Autodesk Inventor part; units mm, degrees
ref_plane "YZ Plane" through (0, 0, 0) normal (1, 0, 0) x (0, 1, 0)
ref_plane "XZ Plane" through (0, 0, 0) normal (0, 1, 0) x (-1, 0, 0)
ref_plane "XY Plane" through (0, 0, 0) normal (0, 0, 1) x (1, 0, 0)
sketch "Sketch1" plane through (0, 0, 0) normal (0, 1, 0) x (-1, 0, 0)
  line L0 (0, 0) -> (-76.2, 0)
  line L1 (-76.2, 0) -> (-76.2, -38.1)
  line L2 (-76.2, -38.1) -> (0, -38.1)
  line L3 (0, -38.1) -> (0, 0)
  dimension "d0" = 76.2
  dimension "d1" = 38.1
extrude "Extrusion1" add sketch "Sketch1" along normal blind 2.54
sketch "Sketch2" plane through (0, 2.54, 0) normal (0, 1, 0) x (1, 0, 0)
  line L0 (0, 0) -> (6.35, 0)
  line L1 (0, 0) -> (76.2, 0)
  line L2 (6.35, 0) -> (6.35, 38.1)
  line L3 (76.2, 38.1) -> (0, 38.1)
  line L4 (6.35, 0) -> (6.35, 9.525)
  line L5 (6.35, 38.1) -> (6.35, 28.575)
  dimension "d4" = 6.35
  dimension "d5" = 9.525
  dimension "d6" = 9.525
hole "Hole1" at (6.35, 2.54, -9.525) at (6.35, 2.54, -28.575) direction (0, -1, 0) diameter 5.08 end through all
fillet "Fillet1" radius 1.27 2 edges at (76.2, 2.54, -19.05) (76.2, 0, -19.05)
fillet "Fillet2" radius 1.27 1 edges at (0, 2.54, -19.05)
properties part number "Cover"
Verification items for the finished model (mm, model axes). Coordinates: 2 decimals unless noted, no trailing zeros. Order: outer loops, then holes, each group sorted by start corner. A loop starts at its lowest first (then second) coordinate and runs counter-clockwise, first axis right, second up. Notation, with made-up numbers: (31.5, 23.5) -> (72.5, 23.5) arc R16 ccw to (72.5, 35.5) -> close; hole circle Ø2 at (-11, -25.75). An arc over 180 degrees is marked (long way). Put each result on its own line as item: value. Start each with the question number.
1) Cross-section at A-A (x = 6.35). Enter the section's corners in (y, z) (3 decimals), plus the area to 3 significant figures.
2) Cross-section at C-C (y = 0.8). Enter the section's corners in (x, z) (3 decimals).
3) Material ranges on L1, parallel to Z at x = 6.35, y = 1.15 (3 decimals); L2, parallel to X at y = 1.35, z = -28.5; L3, parallel to X at y = 1.4, z = -17, recorded low to high.
4) Release check for a two-part mould opening along Z. For faces 1 (the cylindrical face through (7.323, 1.252, -26.229)), 2 (the flat face through (38, 0, -19)), 3 (the flat face through (39, 1, -38.1)), 4 (the flat face through (38, 1, 0)) record: pulls with the +Z half, pulls with the -Z half, needs draft (parallel to the pull), parting line crosses it, or undercut.
Geometry check:
1. outline: (0, -38.1) -> (2.54, -38.1) -> (2.54, -31.115) -> (0, -31.115) -> close; (0, -26.035) -> (2.54, -26.035) -> (2.54, -12.065) -> (0, -12.065) -> close; (0, -6.985) -> (2.54, -6.985) -> (2.54, 0) -> (0, 0) -> close
1. area: 71.0 mm^2
2. outline: (0, -38.1) -> (76.11, -38.1) -> (76.11, 0) -> (0, 0) -> close; hole circle Ø5.08 at (6.35, -28.575); hole circle Ø5.08 at (6.35, -9.525)
3. L1: z = -38.1 to -31.115, -26.035 to -12.065, -6.985 to 0
3. L2: x = 0 to 3.81, 8.89 to 76.2
3. L3: x = 0.01 to 76.19
4. face 1: undercut
4. face 2: needs draft
4. face 3: pulls with the -Z half
4. face 4: pulls with the +Z half
